Could you check a few things on this drawing? It's one solid part, dimensions in mm from its lowest x, y, z. A direction names the side the tool comes from. Round coordinates to 2 decimals unless told otherwise and drop trailing zeros. Write each loop counter-clockwise with the first axis right and the second up, starting at its lowest first coordinate (ties: lowest second). Pieces come first, ordered by that corner, then holes. Notation, with made-up numbers: (-37.5, 75) - (-0.5, 75) arc R35 ccw to (-0.5, 109) - close; hole circle Ø6 at (-27, 0). An arc over 180 degrees is marked (long way). Put each result on its own line as item: value.
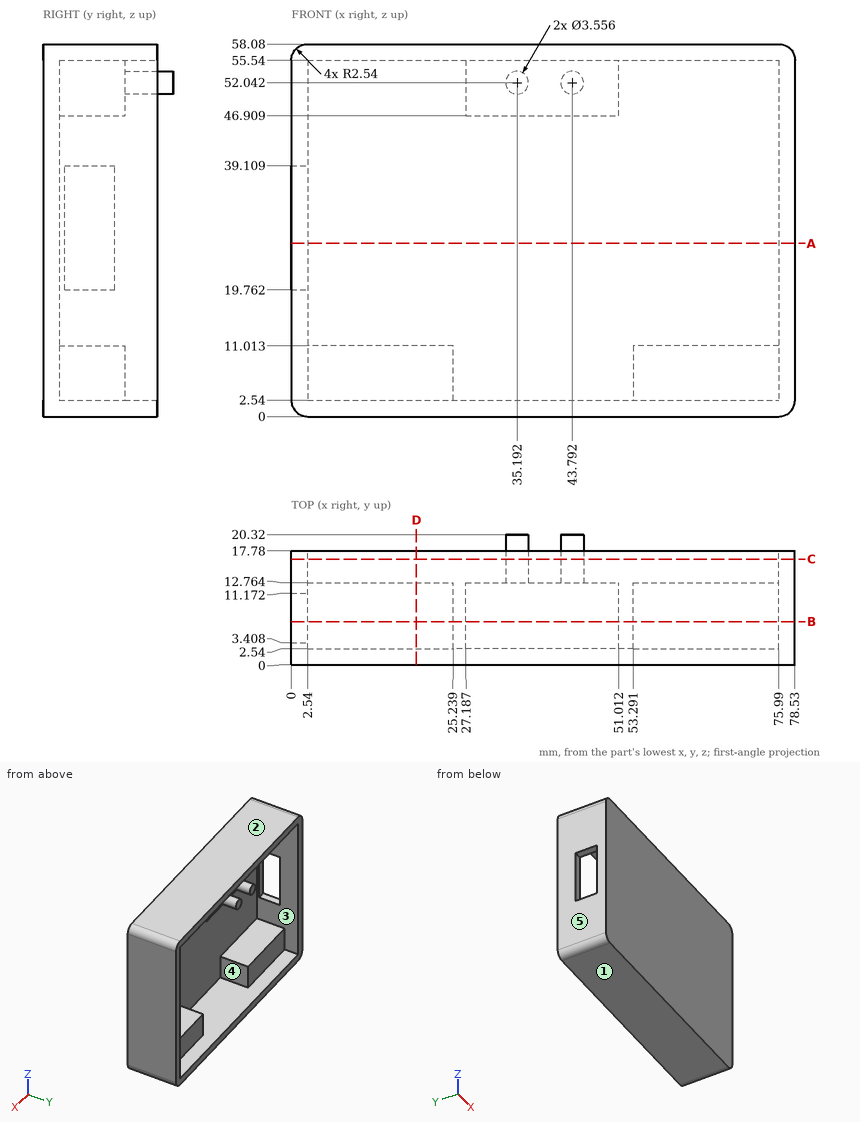
(1) Please list where these lines run through material, in increasing order: probe 1 along Z at (x, y) = (52, 5.75); probe 2 along Z at (x, y) = (28, 11.5); probe 3 along X at (y, z) = (10.75, 40). Write a range as from..to.
Values found:
probe 1: z = 0..2.54, 55.54..58.08
probe 2: z = 0..2.54, 46.91..58.08
probe 3: x = 0..2.54, 75.99..78.53
(2) Imagine slicing it at A-A, the plane z = 27. List the corners of the cut face in (x, y) for me.
Values found:
outline: (0, 0) - (78.53, 0) - (78.53, 17.78) - (75.99, 17.78) - (75.99, 2.54) - (2.54, 2.54) - (2.54, 3.41) - (0, 3.41) - close; (0, 11.17) - (2.54, 11.17) - (2.54, 17.78) - (0, 17.78) - close
(3) Imagine slicing it at B-B, the plane y = 6.75. List the corners of the cut face in (x, z) for me, then the cut area to 3 significant figures.
Values found:
outline: (0, 2.54) arc R2.54 ccw to (2.54, 0) - (75.99, 0) arc R2.54 ccw to (78.53, 2.54) - (78.53, 55.54) arc R2.54 ccw to (75.99, 58.08) - (2.54, 58.08) arc R2.54 ccw to (0, 55.54) - (0, 39.11) - (2.54, 39.11) - (2.54, 55.54) - (27.19, 55.54) - (27.19, 46.91) - (51.01, 46.91) - (51.01, 55.54) - (75.99, 55.54) - (75.99, 11.01) - (53.29, 11.01) - (53.29, 2.54) - (25.24, 2.54) - (25.24, 11.01) - (2.54, 11.01) - (2.54, 19.76) - (0, 19.76) - close
area: 1,200 mm^2
(4) For the marked faces 4 and 5, which set-ups out of +Z, -Z, +X, -X, +Y, -Y let a thin tool reach every point of the face, with its end or its side?
Values found:
face 4: +Y
face 5: +Z, -Z, -X, +Y, -Y
(5) Imagine slicing it at C-C, the plane y = 16.5. List the corners of the cut face in (x, z) for me (1 decimal).
Values found:
outline: (0, 2.5) arc R2.5 ccw to (2.5, 0) - (76, 0) arc R2.5 ccw to (78.5, 2.5) - (78.5, 55.5) arc R2.5 ccw to (76, 58.1) - (2.5, 58.1) arc R2.5 ccw to (0, 55.5) - close; circle Ø3.6 at (35.2, 52); circle Ø3.6 at (43.8, 52); hole (2.5, 2.5) - (76, 2.5) - (76, 55.5) - (2.5, 55.5) - close
(6) I'm going to push flat-ended pins straight in: pin 1 (3 mm diameter, centred on x = 66.5, z = 47, fed in from -Y); pin 2 (0.8 mm diameter, centred on x = 1.5, y = 8, fed in from -Z); pin 3 (5 mm diameter, centred on x = 35.5, z = 27.5, fed in from +Y); pin 4 (7 mm diameter, centred on x = 61, z = 8, fed in from +Y). Where does each tip first touch, or does it pass through?
Values found:
pin 1: stops at y = 0
pin 2: stops at z = 0.08
pin 3: stops at y = 2.54
pin 4: stops at y = 12.76
(7) If we mould it in two halves opening along Z, with no side actions, what happens to the marked faces 1, 2 and 3? For each: pulls with the +Z half, pulls with the -Z half, needs draft (parallel to the pull), parting line crosses it, or undercut.
Values found:
face 1: pulls with the -Z half
face 2: pulls with the +Z half
face 3: undercut
(8) Imagine slicing it at D-D, the plane x = 19.5. List the corners of the cut face in (y, z) for me.
Values found:
outline: (0, 0) - (17.78, 0) - (17.78, 2.54) - (12.76, 2.54) - (12.76, 11.01) - (2.54, 11.01) - (2.54, 55.54) - (17.78, 55.54) - (17.78, 58.08) - (0, 58.08) - close
